```python
from build123d import *

# Parameters (mm, degrees)
SKETCH1_R           = 4
SKETCH1_W           = 42
SKETCH1_H           = 14
SKETCH1_W_2         = 40
BOSS_EXTRUDE1_DEPTH = 10
FILLET1_R           = 7


with BuildPart() as part:
    # Sketch1 → Boss-Extrude1 (new body)
    with BuildSketch(Plane(origin=(0, 0, 0), x_dir=(1, 0, 0), z_dir=(0, 1, 0))):
        with BuildLine():
            Line((-200, 12), (0, 12))
            ThreePointArc((0, 12), (12, 0), (0, -12))
            Line((0, -12), (-200, -12))
            ThreePointArc((-200, -12), (-205.477225575, -10.677078252), (-209.746794345, -7))
            ThreePointArc((-209.746794345, -7), (-212, 0), (-209.746794345, 7))
            ThreePointArc((-209.746794345, 7), (-205.477225575, 10.677078252), (-200, 12))
        make_face()
        with Locations(Location((-200, 0, 0), (0, 0, 270))):
            Circle(SKETCH1_R, mode=Mode.SUBTRACT)
        with Locations(Location((0, 0, 0), (0, 0, 270))):
            Circle(SKETCH1_R, mode=Mode.SUBTRACT)
        with Locations((-167, 0)):
            Rectangle(SKETCH1_W, SKETCH1_H, mode=Mode.SUBTRACT)
        with Locations((-122, 0)):
            Rectangle(SKETCH1_W_2, SKETCH1_H, mode=Mode.SUBTRACT)
        with Locations((-78, 0)):
            Rectangle(SKETCH1_W_2, SKETCH1_H, mode=Mode.SUBTRACT)
        with Locations((-33, 0)):
            Rectangle(SKETCH1_W, SKETCH1_H, mode=Mode.SUBTRACT)
    extrude(amount=BOSS_EXTRUDE1_DEPTH)

    # Fillet1
    fillet1_edges = [part.edges().sort_by_distance(p)[0] for p in [
        (-142, 5, -7),
        (-98, 5, -7),
        (-54, 5, -7),
        (-58, 5, -7),
        (-12, 5, -7),
        (-102, 5, -7),
        (-146, 5, -7),
        (-146, 5, 7),
        (-102, 5, 7),
        (-58, 5, 7),
        (-12, 5, 7),
        (-54, 5, 7),
        (-98, 5, 7),
        (-142, 5, 7),
        (-188, 5, 7),
        (-188, 5, -7),
    ]]
    fillet(fillet1_edges, radius=FILLET1_R - 0.0001)  # a hair under: the kernel refuses the full size


solid = part.part
```
Here's how the part is built. I have some questions about the finished solid (model axes, mm). Give positions to 0.01 mm unless a question says otherwise; leave off trailing zeros. Loops run counter-clockwise (first coordinate to the right, second up) from the corner with the lowest first, then second, coordinate; pieces in that order, holes last. Notation, with made-up numbers: M 88.5,82.25 L 123.5,82.25 A27 ccw 123.5,104.25 Z; hole C -16,36 d5. An arc over 180 degrees is marked long. Use one line per item in the form item = value. Start each with the question number.
Q1. If we section it at A-A (x = -123): Write out the boundary of the cut face in (y, z).
Q2. If we section it at B-B (y = 8.5): State how many separate pieces and enclosed holes the cut face has, then the cut area to 3 significant figures.
Q3. I need wall thicknesses on line 1 along Z through (x, y) = (-83, 1.5); line 2 along X through (y, z) = (1.5, 5); line 3 along X through (y, z) = (5.75, -6). Which ranges of each line are inside material? Lowest first, please.
Q4. If we section it at C-C (z = -10): Write out the boundary of the cut face in (x, y), then the cut area to 3 significant figures.
Q5. Thinking about a two-plate mould opening in Z: for faces 1 (the flat face through (-33, 5, 7)), 2 (the flat face through (-101, 5, -12)), 3 (the flat face through (-98.4, 0, -0.2)), which applies, +Z half, -Z half, draft (parallel to the pull), parting line (faces both ways), or undercut?
Q6. Will these pins go through, and if not, where does the flat tip stop? pin 1 Ø6 at (y, z) = (4, 7.5) entering from -X; pin 2 Ø1.5 at (y, z) = (7.5, -2) entering from +X.
Taken from the geometry:
q1.outline = M 0,-12 L 10,-12 L 10,-7 L 0,-7 Z; M 0,7 L 10,7 L 10,12 L 0,12 Z
q2.separate_pieces = 1
q2.enclosed_holes = 6
q2.area = 3,020 mm^2
q3.line_1 = -12 to -7, 7 to 12
q3.line_2 = -210.91 to -185.9, -148.1 to -139.9, -104.1 to -95.9, -60.1 to -51.9, -14.1 to 10.91
q3.line_3 = -210.39 to -184.61, -149.39 to -138.61, -105.39 to -94.61, -61.39 to -50.61, -15.39 to 10.39
q4.outline = M -206.63,0 L 6.63,0 L 6.63,10 L -206.63,10 Z
q4.area = 2,130 mm^2
q5.face_1 = undercut
q5.face_2 = -Z half
q5.face_3 = draft
q6.pin_1 = -211.12
q6.pin_2 = 11.93
